Autodesk Inventor part; units mm, degrees
ref_plane "mirror-plane" through (17.0812, 13.9062, 0) normal (1, 0, 0) x (0, 0, -1)
ref_plane "YZ Plane" through (0, 0, 0) normal (1, 0, 0) x (0, 1, 0)
ref_plane "XZ Plane" through (0, 0, 0) normal (0, 1, 0) x (-1, 0, 0)
sketch "Sketch1" plane through (0, 0, 0) normal (0, 0, 1) x (1, 0, 0)
  line L0 (-4.0722, -11.1882) -> (-4.7562, -13.0676)
  arc A0 (-4.7562, -13.0676) -> (-4.7562, 13.0676) centre (0, 0) ccw
  line L1 (-4.7562, 13.0676) -> (-4.0722, 11.1882)
  arc A1 (-4.0722, -11.1882) -> (-4.0722, 11.1882) centre (0, 0) ccw
  line L2 (0, 13.9062) -> (20.2562, 13.9062)
  line L3 (20.2562, 13.9062) -> (20.2562, -13.9062)
  line L4 (20.2562, -13.9062) -> (0, -13.9062)
  line L5 (13.9062, 13.9062) -> (13.9063, -13.9062) construction
  line L6 (17.0812, 13.9062) -> (17.0813, -13.9062) construction
  dimension "d0" = 11.9062
  dimension "d1" = 2
  dimension "d2" = 140
  dimension "d3" = 6.35
  dimension "d4" = 3.175
extrude "Extrusion1" add sketch "Sketch1" along normal blind 25.4
ref_plane "mirror-plane" through (17.0812, 13.9062, 0) normal (1, 0, 0) x (0, 0, -1)
equation "\"d1\" = wall"
equation "\"d2\" = angle"
equation "\"d4\" = 0.5 * d3"
equation "\"angle\" = 140deg"
equation "\"wall\" = 2"
properties part number "hook-thingy-base-01"
Work out the finished part from the listing and answer in its coordinate system (mm). A direction names the side the tool comes from. Give positions to 0.01 mm unless a question says otherwise; leave off trailing zeros. Loops run counter-clockwise (first coordinate to the right, second up) from the corner with the lowest first, then second, coordinate; pieces in that order, holes last. Notation, with made-up numbers: (-13, 57) -> (-4, 57) arc R24 ccw to (-4, 85) -> close; hole circle Ø5 at (-17, 56). An arc over 180 degrees is marked (long way). Use a Markdown table: item, result. Add a question column.
1) Each of these flat-tipped pins is pushed along its axis until it touches: P1, Ø6, axis at x = -1, z = 19, coming from the +Y side; P2, Ø4, axis at y = -7, z = 20, coming from the -X side; P3, Ø12, axis at y = 10, z = 12, coming from the -X side; P4, Ø1, axis at y = -9.5, z = 17, coming from the -X side. Where does it stop, or does it pass through?
2) For a pull along Y with two mould halves and no side action, classify faces 3 (the flat face through (-4.42, 12.14, 12.52)), 4 (the cylindrical face through (-2.38, -13.7, 12.52)), 5 (the cylindrical face through (-2.45, 13.69, 12.52)) as +Y half, -Y half, draft (parallel to the pull), parting line (faces both ways), or undercut.
3) The part is cut by section D-D, the plane x = 6.5. Determine the outline of the cut face in (y, z), plus the area to 3 significant figures.
4) The part is cut by section C-C, the plane y = -10.5. Determine the outline of the cut face in (x, z).
5) Consider line 1 along Y through (x, z) = (0, 9.25); line 2 along X through (y, z) = (0, 12.25); line 3 along Y through (x, z) = (-3.25, 19.5). Determine where each line is inside the solid, lowest interval first.
6) The part is cut by section A-A, the plane x = 11.5. Determine the outline of the cut face in (y, z).
7) The part is cut by section B-B, the plane z = 20. Determine the outline of the cut face in (x, y), plus the area to 3 significant figures.
8) Which of the six approach directions +Z, -Z, +X, -X, +Y, -Y give full straight-line access (tool end or side, diameter ignored) to faces 1 (the flat face through (-4.409, -12.115, 12.522)), 2 (the flat face through (20.256, 0, 13))?
Reported:
| question | item | result |
|---|---|---|
| 1 | P1 | stops at y = 13.91 |
| 1 | P2 | stops at x = 7.79 |
| 1 | P3 | stops at x = -4.76 |
| 1 | P4 | stops at x = 6.46 |
| 2 | face 3 | undercut |
| 2 | face 4 | -Y half |
| 2 | face 5 | +Y half |
| 3 | outline | (-13.91, 0) -> (-9.98, 0) -> (-9.98, 25.4) -> (-13.91, 25.4) -> close; (9.98, 0) -> (13.91, 0) -> (13.91, 25.4) -> (9.98, 25.4) -> close |
| 3 | area | 200 mm^2 |
| 4 | outline | (5.61, 0) -> (20.26, 0) -> (20.26, 25.4) -> (5.61, 25.4) -> close |
| 5 | line 1 | y = -13.91 to -11.91, 11.91 to 13.91 |
| 5 | line 2 | x = 11.91 to 20.26 |
| 5 | line 3 | y = -13.52 to -11.45, 11.45 to 13.52 |
| 6 | outline | (-13.91, 0) -> (-3.08, 0) -> (-3.08, 25.4) -> (-13.91, 25.4) -> close; (3.08, 0) -> (13.91, 0) -> (13.91, 25.4) -> (3.08, 25.4) -> close |
| 7 | outline | (-4.76, -13.07) arc R13.91 ccw to (0, -13.91) -> (20.26, -13.91) -> (20.26, 13.91) -> (0, 13.91) arc R13.91 ccw to (-4.76, 13.07) -> (-4.07, 11.19) arc R11.91 cw (long way) to (-4.07, -11.19) -> close |
| 7 | area | 359 mm^2 |
| 8 | face 1 | +Z, -Z, -X |
| 8 | face 2 | +Z, -Z, +X, +Y, -Y |
